Can you work these out from the model? Positions are in its coordinate system, mm. Face numbers are marked on the shaded views. A direction names the side the tool comes from. Give positions to 0.01 mm unless a question says otherwise; leave off trailing zeros. Order: outer loops, then holes, each group sorted by start corner. A loop starts at its lowest first (then second) coordinate and runs counter-clockwise, first axis right, second up. Notation, with made-up numbers: (-9.75, 83.5) - (19.25, 83.5) arc R13 cw to (19.25, 87.5) - close; hole circle Ø5 at (60, -22.5). An arc over 180 degrees is marked (long way). Return JSON: item names as keys, results as strings.
```python
from build123d import *

# Parameters (mm, degrees)
SKETCH1_R           = 28.575
EXTRUDE1_DEPTH      = 27.0002
EXTRUDE1_DEPTH_BACK = 84.1248
CUT_EXTRUDE1_REACH  = 86.125
SKETCH2_R           = 28.575
SKETCH2_R_2         = 23.622
CUT_EXTRUDE3_START  = -27.0002
CUT_EXTRUDE3_DEPTH  = 27.0002
SKETCH18_R          = 9.525
CUT_EXTRUDE4_DEPTH  = 0.254
SKETCH19_R          = 9.525
CUT_EXTRUDE5_DEPTH  = 0.254
CHAMFER1_SIZE       = 0.762
CIRPATTERN1_COUNT   = 4


with BuildPart() as part:
    # Sketch1 → Extrude1 (new body, two sides)
    with BuildSketch(Plane(origin=(0, 0, 0), x_dir=(0, 0, -1), z_dir=(1, 0, 0))) as extrude1_sk:
        Circle(SKETCH1_R)
    extrude(amount=EXTRUDE1_DEPTH)
    extrude(extrude1_sk.sketch, amount=-EXTRUDE1_DEPTH_BACK)

    # Sketch2 → Cut-Extrude1 (cut, up to next)
    with BuildSketch(Plane(origin=(0, 0, 0), x_dir=(0, 0, -1), z_dir=(1, 0, 0)), mode=Mode.PRIVATE) as cut_extrude1_sk1:
        Circle(SKETCH2_R)
        with Locations((0, -4.191)):
            Circle(SKETCH2_R_2, mode=Mode.SUBTRACT)
    cut_extrude1_tool1 = extrude(cut_extrude1_sk1.sketch, amount=-CUT_EXTRUDE1_REACH, mode=Mode.PRIVATE) & part.part
    add(cut_extrude1_tool1.solids().sort_by_distance((0, 0, 27.766777))[0], mode=Mode.SUBTRACT)

    # Sketch4 → Cut-Extrude3 (cut)
    with BuildSketch(Plane.ZY.offset(CUT_EXTRUDE3_START)):
        with BuildLine():
            Line((23.6855, -25.666178421), (23.6855, 17.476089577))
            Line((23.6855, 17.476089577), (0, 31.150919378))
            Line((0, 31.150919378), (-23.6855, 17.476089577))
            Line((-23.6855, 17.476089577), (-23.6855, -25.666178421))
            ThreePointArc((-23.6855, -25.666178421), (0, 34.925), (23.6855, -25.666178421))
        make_face()
    extrude(amount=CUT_EXTRUDE3_DEPTH, mode=Mode.SUBTRACT)

    # Sketch6 → Cut-Revolve2 (revolve, cut)
    with BuildSketch(Plane.XY, mode=Mode.PRIVATE) as cut_revolve2_sk:
        Polygon((0.750392661, 57.15), (27.0002, 11.684), (27.0002, 57.15), align=None)
    revolve(cut_revolve2_sk.sketch.rotate(Axis((-0.562097706, -4.191, 0), (1, 0, 0)), 270), axis=Axis((-0.562097706, -4.191, 0), (1, 0, 0)), mode=Mode.SUBTRACT)  # turned: the seam where the file's is

    # S2D0002 → Cut-Revolve3 (revolve, cut)
    with BuildSketch(Plane(origin=(9.0932, 23.136869081, 13.372742289), x_dir=(0, 0.5, -0.866025404), z_dir=(1, 0, 0))):
        Polygon((0, 0), (6.1849, 0), (5.642306865, -2.5527), (4.9784, -3.216606865), (4.9784, -13.462), (0, -13.462), align=None)
    revolve(axis=Axis((9.0932, 10.895513396, 6.305192289), (0, 0.866025404, 0.5)), mode=Mode.SUBTRACT)

    # Sketch8 → Cut-Revolve4 (revolve, cut)
    with BuildSketch(Plane(origin=(9.0932, 23.136869081, -13.372742289), x_dir=(0, -0.5, -0.866025404), z_dir=(1, 0, 0))):
        Polygon((0, 0), (6.1849, 0), (5.642306865, -2.5527), (4.9784, -3.216606865), (4.9784, -13.462), (0, -13.462), align=None)
    revolve(axis=Axis((9.0932, 10.895513396, -6.305192289), (0, 0.866025404, -0.5)), mode=Mode.SUBTRACT)

    # Sketch18 → Cut-Extrude4 (cut)
    with BuildSketch(Plane(origin=(0, 23.363189534, 13.488743766), x_dir=(1, 0, 0), z_dir=(0, 0.866025404, 0.5))):
        with Locations((9.0932, -0.0127)):
            Circle(SKETCH18_R)
    extrude(amount=-CUT_EXTRUDE4_DEPTH, mode=Mode.SUBTRACT)

    # Sketch19 → Cut-Extrude5 (cut)
    with BuildSketch(Plane(origin=(0, 23.363189534, -13.488743766), x_dir=(1, 0, 0), z_dir=(0, 0.866025404, -0.5))):
        with Locations((9.0932, 0.0127)):
            Circle(SKETCH19_R)
    extrude(amount=-CUT_EXTRUDE5_DEPTH, mode=Mode.SUBTRACT)

    # Sketch10 → Cut-Revolve6 (revolve, cut)
    with BuildSketch(Plane.XY, mode=Mode.PRIVATE) as cut_revolve6_sk:
        Polygon((0, 19.431), (0, 18.415), (-3.302, 18.415), (-4.318, 19.431), align=None)
    revolve(cut_revolve6_sk.sketch.rotate(Axis((-4.5339, -4.191, 0), (1, 0, 0)), 90), axis=Axis((-4.5339, -4.191, 0), (1, 0, 0)), mode=Mode.SUBTRACT)  # turned: the seam where the file's is

    # Sketch12 → Cut-Revolve8 (revolve, cut)
    with BuildSketch(Plane.XY, mode=Mode.PRIVATE) as cut_revolve8_sk:
        Polygon((-84.1248, 19.431), (-84.1248, 18.415), (-81.5848, 18.415), (-80.5688, 19.431), align=None)
    revolve(cut_revolve8_sk.sketch.rotate(Axis((-84.3026, -4.191, 0), (1, 0, 0)), 90), axis=Axis((-84.3026, -4.191, 0), (1, 0, 0)), mode=Mode.SUBTRACT)  # turned: the seam where the file's is

    # Chamfer1
    chamfer1_edges = [part.edges().sort_by_distance(p)[0] for p in [
        (-84.1248, -4.191, -22.606),
    ]]
    chamfer(chamfer1_edges, length=CHAMFER1_SIZE)

    # Sketch13 → Revolve1 (revolve)
    with BuildSketch(Plane(origin=(0, 0, 0), x_dir=(0, -1, 0), z_dir=(0, 0, 1)), mode=Mode.PRIVATE) as revolve1_sk:
        with BuildLine():
            Line((4.191, 27.0002), (4.191, 64.8716))
            Line((4.191, 64.8716), (14.2875, 64.8716))
            ThreePointArc((14.2875, 64.8716), (15.00592049, 64.57402049), (15.3035, 63.8556))
            Line((15.3035, 63.8556), (15.3035, 27.0002))
            Line((15.3035, 27.0002), (4.191, 27.0002))
        make_face()
    revolve(revolve1_sk.sketch.rotate(Axis((25.10663, -4.191, 0), (1, 0, 0)), 270), axis=Axis((25.10663, -4.191, 0), (1, 0, 0)))  # turned: the seam where the file's is

    # S2D0001 → Cut-Revolve9 (revolve, cut)
    with BuildSketch(Plane(origin=(64.8716, -9.9441, 0), x_dir=(0, -1, 0), z_dir=(0, 0, 1)), mode=Mode.PRIVATE) as cut_revolve9_sk:
        Polygon((0, 0), (0, -17.018), (-5.7531, -20.474811227), (-5.7531, 0), align=None)
    revolve(cut_revolve9_sk.sketch.rotate(Axis((43.373048211, -4.191, 0), (1, 0, 0)), 270), axis=Axis((43.373048211, -4.191, 0), (1, 0, 0)), mode=Mode.SUBTRACT)  # turned: the seam where the file's is

    # Sketch16 → Cut-Revolve10 (revolve, cut)
    with BuildSketch(Plane(origin=(60.9092, 3.666724106, -7.857724106), x_dir=(-1, 0, 0), z_dir=(0, -0.707106781, -0.707106781)), mode=Mode.PRIVATE) as cut_revolve10_sk:
        Polygon((0, 0), (2.413, 0), (0, -2.413), align=None)
    cut_revolve10 = revolve(cut_revolve10_sk.sketch.rotate(Axis((60.9092, 0.494324135, -4.685324135), (0, 0.707106781, -0.707106781)), 90), axis=Axis((60.9092, 0.494324135, -4.685324135), (0, 0.707106781, -0.707106781)), mode=Mode.SUBTRACT)  # turned: the seam where the file's is

    # CirPattern1: Cut-Revolve10 ×4 about axis
    cirpattern1_axis = Axis((25.10663, -4.191, 0), (-1, 0, 0))
    for i in range(1, CIRPATTERN1_COUNT):
        add(cut_revolve10.rotate(cirpattern1_axis, i * 360 / CIRPATTERN1_COUNT), mode=Mode.SUBTRACT)


solid = part.part
```
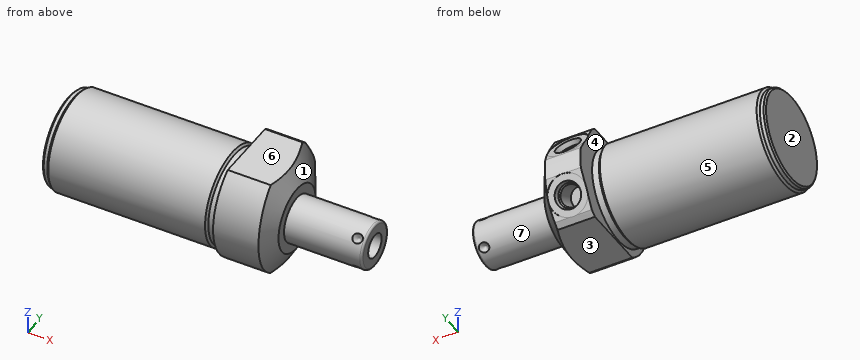
1. For pin 1 Ø2 at (x, z) = (-33.5, 13.5) entering from +Y; pin 2 Ø8 at (x, z) = (-50, 14.5) entering from -Y; pin 3 Ø8 at (x, z) = (42, -0.5) entering from +Y, each with a flat end and sliding along its axis, tell me the tip position at first contact or that it passes through.
Checks:
{"pin 1": "y = 15.85", "pin 2": "y = -25.35", "pin 3": "y = 6.92"}
2. Suppose I cut it at B-B (x = -20). List the corners of the cut face in (y, z) for me, plus the area to 3 significant figures.
Checks:
{"outline": "circle Ø47.24 at (-4.19, 0)", "area": "1,750 mm^2"}
3. On a 3-axis mill with a long thin cutter (end or side, diameter ignored), from which of +Z, -Z, +X, -X, +Y, -Y can I reach the whole of each face in a straight line? I mean the marked faces 5, 6 and 7. Say none if no direction works.
Checks:
{"face 5": "-X", "face 6": "+Z, +X, -X, +Y, -Y", "face 7": "+X"}
4. Thinking about a two-plate mould opening in X: for the marked faces 1, 2, 3 and 4, which applies, +X half, -X half, draft (parallel to the pull), parting line (faces both ways), or undercut?
Checks:
{"face 1": "+X half", "face 2": "-X half", "face 3": "draft", "face 4": "undercut"}
5. If I drill on L1, parallel to Y at x = 55.75, z = 0; L2, parallel to X at y = 18.5, z = 5.5; L3, parallel to X at y = 9.5, z = 4, over which ranges is the centre line in solid material (lowest first)? Write a range as [from, to].
Checks:
{"L1": "[-15.3, -9.94], [1.56, 6.92]", "L2": "[-80.84, -4.04], [0, 6.96], [11.22, 22.69]", "L3": "[-84.12, 27]"}
6. Suppose I cut it at A-A (x = 33.5). List the corners of the cut face in (y, z) for me (1 decimal).
Checks:
{"outline": "circle Ø22.2 at (-4.2, 0)"}
